from build123d import *

# Parameters (mm, degrees)
SKETCH1_W           = 270
SKETCH1_H           = 20
BOSS_EXTRUDE1_DEPTH = 5
SKETCH2_R           = 5
CUT_EXTRUDE1_DEPTH  = 5
SKETCH3_R           = 5
BOSS_EXTRUDE2_DEPTH = 15


with BuildPart() as part:
    # Sketch1 → Boss-Extrude1 (new body)
    with BuildSketch(Plane.XY):
        Rectangle(SKETCH1_W, SKETCH1_H)
    extrude(amount=BOSS_EXTRUDE1_DEPTH)

    # Sketch2 → Cut-Extrude1 (cut)
    with BuildSketch(Plane(origin=(0, 0, 0), x_dir=(-1, 0, 0), z_dir=(0, 0, -1))):
        with Locations((-125, 0)):
            Circle(SKETCH2_R)
    extrude(amount=-CUT_EXTRUDE1_DEPTH, mode=Mode.SUBTRACT)

    # Sketch3 → Boss-Extrude2 (add)
    with BuildSketch(Plane(origin=(0, 0, 0), x_dir=(-1, 0, 0), z_dir=(0, 0, -1))):
        with Locations(Location((125, 0, 0), (0, 0, 180))):
            Circle(SKETCH3_R)
    extrude(amount=BOSS_EXTRUDE2_DEPTH)


solid = part.part
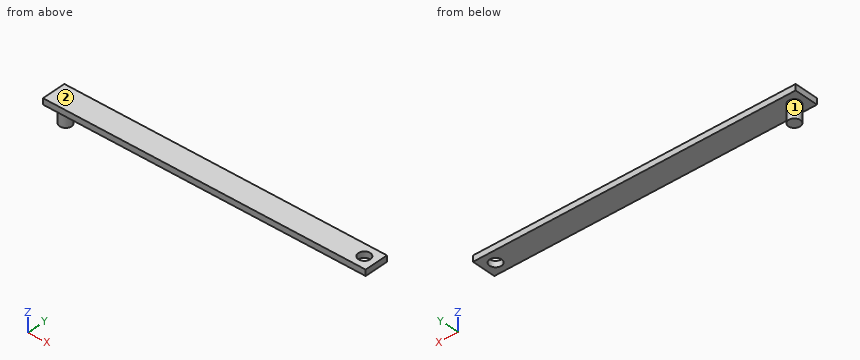
Verification items for the finished model (mm, model axes). Face numbers are marked on the shaded views. A direction names the side the tool comes from. Give positions to 0.01 mm unless a question says otherwise; leave off trailing zeros. Write each loop counter-clockwise with the first axis right and the second up, starting at its lowest first coordinate (ties: lowest second). Pieces come first, ordered by that corner, then holes.
(1) Access from +Z, -Z, +X, -X, +Y, -Y to the whole of each face (thin tool, end or side, straight path). Record for the marked faces 1 and 2.
(2) Cross-section at B-B (y = 0). Enter the section's corners in (x, z).
(3) Cross-section at D-D (z = -12.5). Enter the section's corners in (x, y).
(4) Cross-section at C-C (x = -125). Enter the section's corners in (y, z).
(5) Gauge pin test, flat ends, axial feed: pin 1 (4 mm diameter, centred on x = 21, y = 0.5, fed in from -Z); pin 2 (6 mm diameter, centred on y = -5, z = -5, fed in from -X). Record the tip position at first contact, or that the pin passes through.
(6) Material ranges on line 1 (Y direction, x = 125, z = 1.4); line 2 (Z direction, x = -39.5, y = -4); line 3 (X direction, y = -0.5, z = -10.75), recorded low to high.
(7) Cross-section at A-A (x = 125). Enter the section's corners in (y, z).
Worked out:
1. face 1: -Z
1. face 2: +Z, +X, -X, +Y, -Y
2. outline: (-135, 0) - (-130, 0) - (-130, -15) - (-120, -15) - (-120, 0) - (120, 0) - (120, 5) - (-135, 5) - close; (130, 0) - (135, 0) - (135, 5) - (130, 5) - close
3. outline: circle Ø10 at (-125, 0)
4. outline: (-10, 0) - (-5, 0) - (-5, -15) - (5, -15) - (5, 0) - (10, 0) - (10, 5) - (-10, 5) - close
5. pin 1: stops at z = 0
5. pin 2: stops at x = -129.58
6. line 1: y = -10 to -5, 5 to 10
6. line 2: z = 0 to 5
6. line 3: x = -129.97 to -120.03
7. outline: (-10, 0) - (-5, 0) - (-5, 5) - (-10, 5) - close; (5, 0) - (10, 0) - (10, 5) - (5, 5) - close
